The listing builds one solid part. Answer for the finished solid, in the listing's coordinates (mm). A direction names the side the tool comes from. Round coordinates to 2 decimals unless told otherwise and drop trailing zeros. Loops run counter-clockwise (first coordinate to the right, second up) from the corner with the lowest first, then second, coordinate; pieces in that order, holes last. Notation, with made-up numbers: M 77.5,17.25 L 110.5,17.25 A27 cw 110.5,34.25 Z; hole C 16.5,2 d5. An arc over 180 degrees is marked long. Put each result on its own line as item: value. Start each with the question number.
(1) Straight lines are drawn through the part: line 1 (Y direction, x = 0, z = -1.5) (3 decimals); line 2 (X direction, y = -3, z = -3); line 3 (X direction, y = 1.5, z = 5.25). For each, find the intervals that lie inside material, in ascending order.
(2) Section A-A, the plane x = 0 is taken. Determine the outline of the cut face in (y, z) (3 decimals), then the cut area to 3 significant figures.
(3) Which of the six approach directions +Z, -Z, +X, -X, +Y, -Y give full straight-line access (tool end or side, diameter ignored) to faces 4 (the face through (48.172, -0.778, -6.803)), 5 (the face through (-53.34, 4, 0)), 6 (the face through (4, 5.715, 0))?
(4) Determine the mould class of faces 1 (the face through (-63.5, 0, 0)), 2 (the face through (63.5, 0, 0)), 3 (the face through (52.46, -0.035, 6.217)) for opening direction X: released by +X, released by -X, zero draft, split by the parting line, or undercut.
(5) A flat-ended cylindrical pin translates along its axis: P1, Ø1.9, axis at x = -56, z = 2.5, coming from the +Y side (3 decimals). Find the tip coordinate at first contact, or state that the pin passes through.
```python
from build123d import *

# Parameters (mm, degrees)
SKETCH1_W           = 127
SKETCH1_H           = 11.43
BOSS_EXTRUDE1_DEPTH = 8.128
SKETCH6_W           = 3.81
SKETCH6_H           = 2.54
CUT_EXTRUDE1_DEPTH  = 16.256
SKETCH12_R          = 3.81
CUT_EXTRUDE2_DEPTH  = 16.256
SKETCH14_R          = 6.223
CUT_EXTRUDE3_DEPTH  = 25.4
CUT_EXTRUDE4_REACH  = 18.256
SKETCH17_R          = 2.032


with BuildPart() as part:
    # Sketch1 → Boss-Extrude1 (new body, symmetric)
    with BuildSketch(Plane.XY):
        Rectangle(SKETCH1_W, SKETCH1_H)
    extrude(amount=BOSS_EXTRUDE1_DEPTH, both=True)

    # Sketch6 → Cut-Extrude1 (cut)
    with BuildSketch(Plane.XY.offset(8.128)):
        with Locations((-55.245, 4.445)):
            Rectangle(SKETCH6_W, SKETCH6_H)
    extrude(amount=-CUT_EXTRUDE1_DEPTH, mode=Mode.SUBTRACT)

    # Sketch12 → Cut-Extrude2 (cut)
    with BuildSketch(Plane.XY.offset(8.128)):
        Circle(SKETCH12_R)
    extrude(amount=-CUT_EXTRUDE2_DEPTH, mode=Mode.SUBTRACT)

    # Sketch14 → Cut-Extrude3 (cut)
    with BuildSketch(Plane(origin=(2.89208185, -16.401811214, 0), x_dir=(0, 0, -1), z_dir=(0.173648178, -0.984807753, 0))):
        with Locations((0, 51.382892981)):
            Circle(SKETCH14_R)
    extrude(amount=-CUT_EXTRUDE3_DEPTH, mode=Mode.SUBTRACT)

    # Sketch17 → Cut-Extrude4 (cut, up to next)
    with BuildSketch(Plane(origin=(0, 0, -8.128), x_dir=(-1, 0, 0), z_dir=(0, 0, -1)), mode=Mode.PRIVATE) as cut_extrude4_sk1:
        with Locations((-50.048620668, 0)):
            Circle(SKETCH17_R)
    cut_extrude4_tool1 = extrude(cut_extrude4_sk1.sketch, amount=-CUT_EXTRUDE4_REACH, mode=Mode.PRIVATE) & part.part
    add(cut_extrude4_tool1.solids().sort_by_distance((50.048621, 0, -8.128))[0], mode=Mode.SUBTRACT)


solid = part.part
```
Recorded:
1. line 1: y = -5.715 to -3.81, 3.81 to 5.715
1. line 2: x = -63.5 to -2.35, 2.35 to 47.17, 58.24 to 63.5
1. line 3: x = -63.5 to -3.5, 3.5 to 48.52, 55.3 to 63.5
2. outline: M -5.715,-8.128 L -3.81,-8.128 L -3.81,8.128 L -5.715,8.128 Z; M 3.81,-8.128 L 5.715,-8.128 L 5.715,8.128 L 3.81,8.128 Z
2. area: 61.9 mm²
3. face 4: -Z
3. face 5: +Z, -Z, +Y
3. face 6: +Z, -Z, +X, -X, +Y
4. face 1: released by -X
4. face 2: released by +X
4. face 3: undercut
5. P1: stops at y = 3.175
